Verification items for the finished model (mm, model axes). A direction names the side the tool comes from. Give positions to 0.01 mm unless a question says otherwise; leave off trailing zeros. Order: outer loops, then holes, each group sorted by start corner. A loop starts at its lowest first (then second) coordinate and runs counter-clockwise, first axis right, second up. Notation, with made-up numbers: (45.25, -15) -> (90.25, -15) arc R13 ccw to (90.25, 3) -> close; hole circle Ø1 at (67, 64.5). An arc over 180 degrees is marked (long way). One line per question, with ' | ' between items. Start each with the question number.
Q1. Mould release check, pull along Y, two halves, no side actions. Record for faces 1 (the cylindrical face through (41.359, -12.165, -13.267)), 2 (the flat face through (6.474, 1.2, -1.2)), 3 (the flat face through (10.474, 0, 7)), 4 (the cylindrical face through (68.22, 10.65, -13.89)): released by +Y, released by -Y, zero draft, split by the parting line, or undercut.
Q2. Access from +Z, -Z, +X, -X, +Y, -Y to the whole of each face (thin tool, end or side, straight path). Record for faces 5 (the flat face through (70.474, 1.2, 1.2)), 6 (the cylindrical face through (15.4, 0, -11.5)), 7 (the cylindrical face through (38.92, -0.45, 1.43)).
Q3. Go/stop test with flat-tipped pins: pin 1 (6 mm diameter, centred on y = -2.5, z = 2.5, fed in from +X); pin 2 (1.5 mm diameter, centred on x = 33.5, y = -10, fed in from -Z); pin 3 (6 mm diameter, centred on x = 31, z = -9, fed in from -Y); pin 4 (1.2 mm diameter, centred on y = 0, z = -12.5, fed in from +X). Record where each tip stops, or that it passes through.
Q4. Material ranges on probe 1 along Y at (x, z) = (32, 0); probe 2 along Y at (x, z) = (70.7, 0); probe 3 along X at (y, z) = (-5.5, -6.5), recorded low to high. Write a range as [from, to].
Q5. Section check A-A on x = 39. Record the cut outline in (y, z), plus the area to 3 significant figures.
from build123d import *

# Parameters (mm, degrees)
CONG_1_R                = 0.25
CONG_2_R                = 3
ESQUISSE2_R             = 1
ENL_V_MAT_EXTRU_1_DEPTH = 10


with BuildPart() as part:
    # Esquisse1 → Révolution1 (revolve)
    with BuildSketch(Plane.XY, mode=Mode.PRIVATE) as r_volution1_sk:
        Polygon((15.571393841, 1.5), (6.47350081, 1.5), (6.47350081, 6), (5.97350081, 6), (5.97350081, 6.5), (10.47350081, 6.5), (10.47350081, 18), (68.47350081, 18), (68.47350081, 17.502971724), (67.97350081, 17.502971724), (67.97350081, 6.5), (70.97350081, 6.5), (70.97350081, 6), (70.47350081, 6), (70.47350081, 1.5), align=None)
    revolve(r_volution1_sk.sketch.rotate(Axis((0, 0, 0), (1, 0, 0)), 90), axis=Axis((0, 0, 0), (1, 0, 0)))

    # Congé1
    cong_1_edges = [part.edges().sort_by_distance(p)[0] for p in [
        (70.97350081, 0, -6.5),
        (10.47350081, 0, -6.5),
        (5.97350081, 0, -6.5),
    ]]
    fillet(cong_1_edges, radius=CONG_1_R)

    # Congé2
    cong_2_edges = [part.edges().sort_by_distance(p)[0] for p in [
        (10.47350081, 0, -18),
    ]]
    fillet(cong_2_edges, radius=CONG_2_R)

    # Esquisse2 → Enlèv. mat.-Extru.1 (cut)
    with BuildSketch(Plane.ZY.offset(-10.47350081)):
        with Locations((12.5, 0)):
            Circle(ESQUISSE2_R)
        with Locations(Location((-12.5, 0, 0), (0, 0, 180))):
            Circle(ESQUISSE2_R)
    extrude(amount=-ENL_V_MAT_EXTRU_1_DEPTH, mode=Mode.SUBTRACT)


solid = part.part
Filled in:
1) face 1: split by the parting line | face 2: undercut | face 3: zero draft | face 4: undercut
2) face 5: +X | face 6: -X | face 7: +X, -X
3) pin 1: x = 70.97 | pin 2: z = -15.44 | pin 3: y = -16.97 | pin 4: x = 67.97
4) probe 1: [-18, -1.5], [1.5, 18] | probe 2: [-6.5, -6], [6, 6.5] | probe 3: [10.47, 67.97]
5) outline: circle Ø36 at (0, 0); hole circle Ø3 at (0, 0) | area: 1,010 mm²
